Autodesk Inventor part; units mm, degrees
ref_plane "YZ Plane" through (0, 0, 0) normal (1, 0, 0) x (0, 1, 0)
ref_plane "XZ Plane" through (0, 0, 0) normal (0, 1, 0) x (-1, 0, 0)
ref_plane "XY Plane" through (0, 0, 0) normal (0, 0, 1) x (1, 0, 0)
sketch "Sketch1" plane through (0, 0, 0) normal (0, 0, 1) x (1, 0, 0)
  line L0 (7.9375, 0) -> (3.9688, -6.8741)
  line L1 (3.9688, -6.8741) -> (-3.9687, -6.8741)
  line L2 (-3.9687, -6.8741) -> (-7.9375, 0)
  line L3 (-7.9375, 0) -> (-3.9688, 6.8741)
  line L4 (-3.9688, 6.8741) -> (3.9688, 6.8741)
  line L5 (3.9688, 6.8741) -> (7.9375, 0)
  point P0 (0, 0)
  point P1 (0, 0)
  dimension "d0" = 15.875
extrude "Extrusion1" add sketch "Sketch1" along normal blind 5.08
sketch "Sketch2" plane through (0, 0, 5.08) normal (0, 0, 1) x (1, 0, 0)
  circle A0 centre (0, 0) radius 3.81
  dimension "d3" = 7.62
extrude "Extrusion2" add sketch "Sketch2" along normal blind 16.002
thread "Thread1"
chamfer "Chamfer1" distance 0.3175 angle 45 1 edges at (-3.81, 0, 21.082)
fillet "Fillet1" radius 0.3175 12 edges at (5.9531, 3.437, 5.08) (0, 6.8741, 5.08) (-5.9531, 3.437, 5.08) (-5.9531, -3.437, 5.08) (0, -6.8741, 5.08) (5.9531, -3.437, 5.08) (5.9531, -3.437, 0) (0, -6.8741, 0) (-5.9531, -3.437, 0) (-5.9531, 3.437, 0) (0, 6.8741, 0) (5.9531, 3.437, 0)
properties part number "Small Bolt"
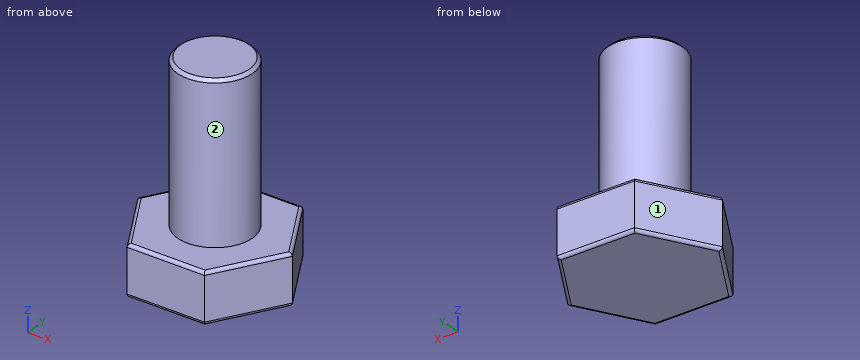
Check sheet for the modelled part. Datum: model origin and axes. Units: mm. Face numbers are marked on the shaded views. A direction names the side the tool comes from. Give positions to 0.01 mm unless a question says otherwise; leave off trailing zeros. Write each loop counter-clockwise with the first axis right and the second up, starting at its lowest first coordinate (ties: lowest second). Pieces come first, ordered by that corner, then holes.
Item 1: Cross-section at B-B (z = 5.5). Enter the section's corners in (x, y).
Item 2: Access from +Z, -Z, +X, -X, +Y, -Y to the whole of each face (thin tool, end or side, straight path). Record for the marked faces 1 and 2.
Item 3: Cross-section at A-A (x = 0). Enter the section's corners in (y, z) (1 decimal).
Item 4: Gauge pin test, flat ends, axial feed: pin 1 (1.5 mm diameter, centred on y = -4, z = 7.5, fed in from +X); pin 2 (3 mm diameter, centred on y = 0.5, z = 8.5, fed in from -X); pin 3 (2 mm diameter, centred on y = -4.5, z = 7, fed in from +X). Record the tip position at first contact, or that the pin passes through.
Item 5: Scan lines: L1, parallel to Z at x = 6, y = -2.5; L2, parallel to Y at x = 5.75, z = 3; L3, parallel to X at y = 1, z = 14.5. Record each from-to range of solid material in increasing order.
Report:
1. outline: circle Ø7.62 at (0, 0)
2. face 1: +Z, -Z, -X, +Y
2. face 2: +Z
3. outline: (-6.9, 0.3) arc R0.3 ccw to (-6.6, 0) - (6.6, 0) arc R0.3 ccw to (6.9, 0.3) - (6.9, 4.8) arc R0.3 ccw to (6.6, 5.1) - (3.8, 5.1) - (3.8, 20.8) - (3.5, 21.1) - (-3.5, 21.1) - (-3.8, 20.8) - (-3.8, 5.1) - (-6.6, 5.1) arc R0.3 ccw to (-6.9, 4.8) - close
4. pin 1: stops at x = 1.99
4. pin 2: stops at x = -3.81
4. pin 3: stops at x = 1.51
5. L1: z = 0 to 5.08
5. L2: y = -3.79 to 3.79
5. L3: x = -3.68 to 3.68
